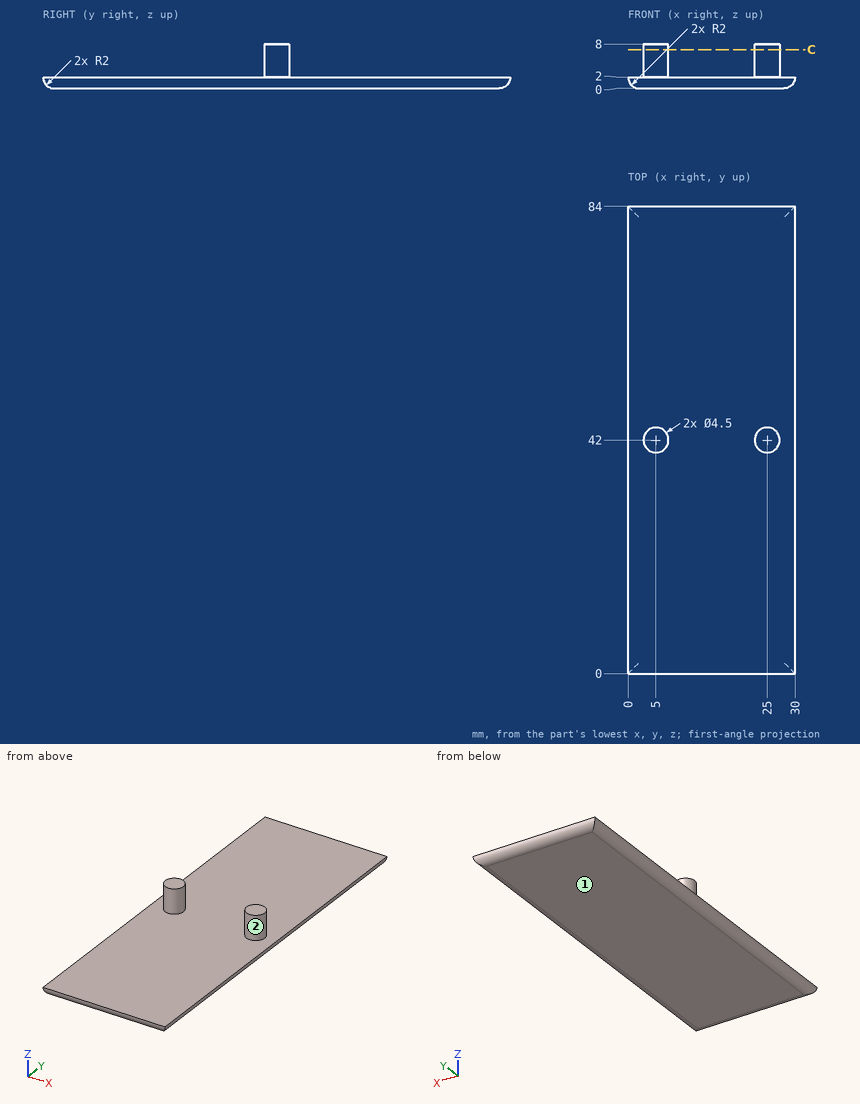
Study the drawing (mm; zero at the part's minimum x, y, z) and answer. Give positions to 0.01 mm unless a question says otherwise; leave off trailing zeros. Write each loop counter-clockwise with the first axis right and the second up, starting at its lowest first coordinate (ties: lowest second). Pieces come first, ordered by that corner, then holes. Notation, with made-up numbers: (-5, 53.5) - (32, 53.5) arc R14 cw to (32, 70.5) - close; hole circle Ø1 at (74.25, 50). An arc over 180 degrees is marked (long way). One line per question, with ' | ' between items. Start each with the question number.
1. Straight lines are drawn through the part: line 1 (X direction, y = 27.5, z = 1.75); line 2 (Z direction, x = 12.75, y = 54); line 3 (Y direction, x = 3, z = 1.75). For each, find the intervals that lie inside material, in ascending order.
2. Determine the mould class of the marked faces 1 and 2 for opening direction X: +X half, -X half, draft (parallel to the pull), parting line (faces both ways), or undercut.
3. Given P1, Ø12, axis at x = 6, y = 68.5, coming from the +Z side, flat-ended and moving along its own axis, determine where the tip first touches the part or whether it passes through.
4. Section C-C, the plane z = 7 is taken. Determine the outline of the cut face in (x, y), then the cut area to 3 significant figures.
Result:
1) line 1: x = 0.02 to 29.98 | line 2: z = 0 to 2 | line 3: y = 0.02 to 83.98
2) face 1: draft | face 2: undercut
3) P1: stops at z = 2
4) outline: circle Ø4.5 at (5, 42); circle Ø4.5 at (25, 42) | area: 31.8 mm2
